Source: CAD feature listing. Evaluate the final solid. Frame: model axes, mm. A direction names the side the tool comes from. Give positions to 0.01 mm unless a question says otherwise; leave off trailing zeros. Loops run counter-clockwise (first coordinate to the right, second up) from the corner with the lowest first, then second, coordinate; pieces in that order, holes last.
```python
from build123d import *

# Parameters (mm, degrees)
EXTRUDE_1_DEPTH     = 30
SKETCH_2_R          = 3
CUT_EXTRUDE_1_DEPTH = 87
SKETCH_3_W          = 50
SKETCH_3_H          = 85.391611022
CUT_EXTRUDE_2_DEPTH = 87
SKETCH_4_R          = 3
EXTRUDE_2_DEPTH     = 56
FILLET_1_R          = 15
FILLET_2_R          = 15
CUT_EXTRUDE_3_DEPTH = 85


with BuildPart() as part:
    # 草图1 → 凸台-拉伸1 (new body)
    with BuildSketch(Plane.XY):
        with BuildLine():
            Line((30, -95.393920142), (30, 70))
            Line((30, 70), (-30, 70))
            Line((-30, 70), (-30, -95.393920142))
            ThreePointArc((-30, -95.393920142), (0, -100), (30, -95.393920142))
        make_face()
    extrude(amount=EXTRUDE_1_DEPTH)

    # 草图2 → 切除-拉伸1 (cut)
    with BuildSketch(Plane(origin=(30, 0, 0), x_dir=(0, 0, -1), z_dir=(1, 0, 0))):
        with Locations((-15, -85.393920142)):
            Circle(SKETCH_2_R)
    extrude(amount=-CUT_EXTRUDE_1_DEPTH, mode=Mode.SUBTRACT)

    # 草图3 → 切除-拉伸2 (cut)
    with BuildSketch(Plane.XY.offset(30)):
        with Locations((0, 27.304194489)):
            Rectangle(SKETCH_3_W, SKETCH_3_H)
    extrude(amount=-CUT_EXTRUDE_2_DEPTH, mode=Mode.SUBTRACT)

    # 草图4 → 凸台-拉伸2 (add)
    with BuildSketch(Plane(origin=(30, 0, 0), x_dir=(0, 0, -1), z_dir=(1, 0, 0))):
        with Locations((-15, 55)):
            Circle(SKETCH_4_R)
    extrude(amount=-EXTRUDE_2_DEPTH)

    # 圆角1
    fillet_1_edges = [part.edges().sort_by_distance(p)[0] for p in [
        (0, -100, 30),
    ]]
    fillet(fillet_1_edges, radius=FILLET_1_R)

    # 圆角2
    fillet_2_edges = [part.edges().sort_by_distance(p)[0] for p in [
        (0, -100, 0),
    ]]
    fillet(fillet_2_edges, radius=FILLET_2_R - 0.0001)  # a hair under: the kernel refuses the full size

    # 草图5 → 切除-拉伸3 (cut)
    with BuildSketch(Plane.ZY.offset(30)):
        with BuildLine():
            Line((30, 55), (48.391224998, 55))
            Line((48.391224998, 55), (48.391224998, 76.557809972))
            Line((48.391224998, 76.557809972), (-10.714250248, 76.557809972))
            Line((-10.714250248, 76.557809972), (-10.714250248, 55))
            Line((-10.714250248, 55), (0, 55))
            ThreePointArc((0, 55), (15, 70), (30, 55))
        make_face()
    extrude(amount=-CUT_EXTRUDE_3_DEPTH, mode=Mode.SUBTRACT)


solid = part.part
```
(1) First-contact query: pin 1 (6 mm diameter, centred on x = 6.5, z = 19, fed in from +Y); pin 2 (15 mm diameter, centred on x = 4.5, z = 17, fed in from +Y); pin 3 (2 mm diameter, centred on x = -19.5, z = 20, fed in from +Y). Flat tips, straight axial feed; report the tip coordinate or a pass-through.
A:
pin 1: stops at y = 57.83
pin 2: stops at y = 58
pin 3: stops at y = -15.39
(2) Section D-D, the plane z = 3. Return the cut outline in (x, y).
A:
outline: (-30, -89.08) arc R94 ccw to (30, -89.08) - (30, 64) - (25, 64) - (25, -15.39) - (-25, -15.39) - (-25, 64) - (-30, 64) - close
(3) Ray query, line 1 along X through (y, z) = (40, 26.5); line 2 along Y through (x, z) = (3.5, 15); line 3 along Y through (x, z) = (14, 15). Return the intervals inside material, ascending.
A:
line 1: x = -30 to -25, 25 to 30
line 2: y = -99.94 to -88.39, -82.39 to -15.39, 52 to 58
line 3: y = -99.02 to -88.39, -82.39 to -15.39, 52 to 58
(4) Section C-C, the plane x = 4.5. Count the separate pieces of the cut face and the enclosed holes in it, then the cut area to 3 significant figures.
A:
separate pieces: 2
enclosed holes: 1
area: 2,440 mm2
(5) Section B-B, the plane z = 13.5. Return the cut outline in (x, y).
A:
outline: (-30, -95.32) arc R99.92 ccw to (30, -95.32) - (30, -87.99) - (-30, -87.99) - close; (-30, -82.8) - (30, -82.8) - (30, 69.92) - (25, 69.92) - (25, 57.6) - (-25, 57.6) - (-25, 69.92) - (-30, 69.92) - close; hole (-25, -15.39) - (25, -15.39) - (25, 52.4) - (-25, 52.4) - close
(6) Reachability of faces 4 (the cylindrical face through (0, 58, 15)), 5 (the cylindrical face through (27, 70, 15)) from +Z, -Z, +X, -X, +Y, -Y: full face, straight path, thin tool, end or side. Return the list, or none.
A:
face 4: none
face 5: +X, -X, +Y
(7) Section A-A, the plane y = 2. Return the cut outline in (x, z).
A:
outline: (-30, 0) - (-25, 0) - (-25, 30) - (-30, 30) - close; (25, 0) - (30, 0) - (30, 30) - (25, 30) - close
(8) Mould query, pull axis X, two halves, no side actions, for faces 1 (the flat face through (0, -15.392, 15)), 2 (the flat face through (30, -12, 15)), 3 (the cylindrical face through (0.42, -88.323, 15.65)). Classes: pulls with the +X half, pulls with the -X half, needs draft (parallel to the pull), parting line crosses it, or undercut.
A:
face 1: undercut
face 2: pulls with the +X half
face 3: needs draft
